from build123d import *

# Parameters (mm, degrees)
SKETCH2_R          = 1.525
CUT_EXTRUDE1_DEPTH = 12.61787595


with BuildPart() as part:
    # Sketch1 → Revolve1 (revolve)
    with BuildSketch(Plane.XY, mode=Mode.PRIVATE) as revolve1_sk:
        Polygon((-1.68761801, 2.864823944), (-0.83761801, 2.864823944), (0.28238199, 2.064823944), (1.40238199, 2.864823944), (2.25238199, 2.864823944), (2.25238199, -3.135176056), (-1.68761801, -3.135176056), align=None)
    revolve(revolve1_sk.sketch.rotate(Axis((-1.68761801, -3.135176056, 0), (1, 0, 0)), 90), axis=Axis((-1.68761801, -3.135176056, 0), (1, 0, 0)))

    # Sketch2 → Cut-Extrude1 (cut, through all)
    with BuildSketch(Plane.ZY.offset(1.68761801)):
        with Locations((0, -3.135176056)):
            Circle(SKETCH2_R)
    extrude(amount=-CUT_EXTRUDE1_DEPTH, mode=Mode.SUBTRACT)


solid = part.part
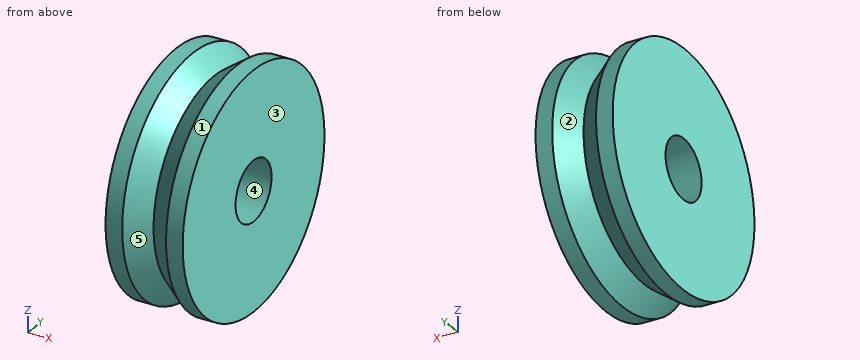
Design review of the part built by this model. Coordinates are the model's own, in mm. Face numbers are marked on the shaded views. A direction names the side the tool comes from. Coordinates: 2 decimals unless noted, no trailing zeros. Order: outer loops, then holes, each group sorted by start corner. A loop starts at its lowest first (then second) coordinate and runs counter-clockwise, first axis right, second up.
Item 1: Take a section at B-B, the plane x = 1.75. Write out the cut boundary in (y, z) (3 decimals).
Item 2: For pin 1 Ø2 at (x, z) = (-0.5, -1.5) entering from -Y, flat-tipped, find the tip position at first contact; note if it passes through.
Item 3: For the marked faces 4 and 5, list the 3-axis set-ups (+Z, -Z, +X, -X, +Y, -Y) from which the entire face can be reached by the end or side of a thin tool; tool diameter is ignored.
Item 4: The part is to be moulded in two halves that separate along X. For the marked faces 1, 2 and 3, say which applies: pulls with the +X half, pulls with the -X half, needs draft (parallel to the pull), parting line crosses it, or undercut.
Item 5: Take a section at A-A, the plane z = 0. Write out the cut boundary in (x, y), then the cut area to 3 significant figures.
Item 6: Take a section at C-C, the plane x = 0.5. Write out the cut boundary in (y, z) (3 decimals).
Item 7: For line 1 (Y direction, x = -0.85, z = 0); line 2 (Z direction, x = 1.2, y = -3.75); line 3 (Y direction, x = -0.7, z = 0.75), list the stretches that pass through material, from the lowest coordinate up.
The answers:
1. outline: circle Ø12 at (-3.135, 0); hole circle Ø3.05 at (-3.135, 0)
2. pin 1: stops at y = -9.11
3. face 4: +X, -X
3. face 5: none
4. face 1: needs draft
4. face 2: undercut
4. face 3: pulls with the +X half
5. outline: (-1.69, -9.14) - (-0.84, -9.14) - (0.28, -8.34) - (1.4, -9.14) - (2.25, -9.14) - (2.25, -4.66) - (-1.69, -4.66) - close; (-1.69, -1.61) - (2.25, -1.61) - (2.25, 2.86) - (1.4, 2.86) - (0.28, 2.06) - (-0.84, 2.86) - (-1.69, 2.86) - close
5. area: 33.5 mm2
6. outline: circle Ø10.711 at (-3.135, 0); hole circle Ø3.05 at (-3.135, 0)
7. line 1: y = -9.14 to -4.66, -1.61 to 2.86
7. line 2: z = -5.82 to -1.4, 1.4 to 5.82
7. line 3: y = -8.99 to -4.46, -1.81 to 2.72
